Here's how the part is built. I have some questions about the finished solid (model axes, mm). A direction names the side the tool comes from. Round coordinates to 2 decimals unless told otherwise and drop trailing zeros. Write each loop counter-clockwise with the first axis right and the second up, starting at its lowest first coordinate (ties: lowest second). Pieces come first, ordered by that corner, then holes. Notation, with made-up numbers: (-15, 80) -> (10, 80) arc R20 ccw to (10, 107) -> close; hole circle Ø2 at (27.25, -31). An arc over 180 degrees is marked (long way). Answer as CSV lines item,"result".
from build123d import *

# Parameters (mm, degrees)
SKETCH1_W               = 1100
SKETCH1_H               = 670
BOSS_EXTRUDE1_DEPTH     = 15
SKETCH2_W               = 30
SKETCH2_H               = 30
BOSS_EXTRUDE2_DEPTH     = 725
MIRROR2_COPY_1_SKETCH_W = 30
MIRROR2_COPY_1_SKETCH_H = 30
MIRROR2_COPY_1_DEPTH    = 725
BOSS_EXTRUDE3_REACH     = 1112.808
SKETCH3_W               = 20
SKETCH3_H               = 40
BOSS_EXTRUDE4_REACH     = 1334.794
SKETCH4_W               = 20
SKETCH4_H               = 40


with BuildPart() as part:
    # Sketch1 → Boss-Extrude1 (new body)
    with BuildSketch(Plane(origin=(0, 0, 0), x_dir=(1, 0, 0), z_dir=(0, 1, 0))):
        Rectangle(SKETCH1_W, SKETCH1_H)
    extrude(amount=BOSS_EXTRUDE1_DEPTH)

    # Sketch2 → Boss-Extrude2 (add)
    with BuildSketch(Plane(origin=(0, 0, 0), x_dir=(1, 0, 0), z_dir=(0, 1, 0))):
        with Locations((-532, -317)):
            Rectangle(SKETCH2_W, SKETCH2_H)
    boss_extrude2 = extrude(amount=-BOSS_EXTRUDE2_DEPTH)

    # Mirror1: Boss-Extrude2 across plane
    add(boss_extrude2.mirror(Plane.XY))

    # Mirror2: Boss-Extrude2 across plane
    add(boss_extrude2.mirror(Plane(origin=(0, 0, 0), x_dir=(0, 0, 1), z_dir=(1, 0, 0))))

    # Mirror2 copy 1 sketch → Mirror2 copy 1 (add)
    with BuildSketch(Plane(origin=(0, 0, 0), x_dir=(-1, 0, 0), z_dir=(0, 1, 0))):
        with Locations((-532, -317)):
            Rectangle(MIRROR2_COPY_1_SKETCH_W, MIRROR2_COPY_1_SKETCH_H)
    extrude(amount=-MIRROR2_COPY_1_DEPTH)

    # Sketch3 → Boss-Extrude3 (add, up to next)
    with BuildSketch(Plane.XY.offset(-302), mode=Mode.PRIVATE) as boss_extrude3_sk1:
        with Locations((-527, -20)):
            Rectangle(SKETCH3_W, SKETCH3_H)
    boss_extrude3_tool1 = extrude(boss_extrude3_sk1.sketch, amount=BOSS_EXTRUDE3_REACH, mode=Mode.PRIVATE) - part.part
    boss_extrude3 = boss_extrude3_tool1.solids().sort_by_distance((-527, -20, -302))[0]
    add(boss_extrude3)

    # Mirror3: Boss-Extrude3 across plane
    add(boss_extrude3.mirror(Plane(origin=(0, 0, 0), x_dir=(0, 0, 1), z_dir=(1, 0, 0))))

    # Sketch4 → Boss-Extrude4 (add, up to next)
    with BuildSketch(Plane(origin=(-517, 0, 0), x_dir=(0, 0, -1), z_dir=(1, 0, 0)), mode=Mode.PRIVATE) as boss_extrude4_sk1:
        with Locations((-312, -20)):
            Rectangle(SKETCH4_W, SKETCH4_H)
    boss_extrude4_tool1 = extrude(boss_extrude4_sk1.sketch, amount=BOSS_EXTRUDE4_REACH, mode=Mode.PRIVATE) - part.part
    boss_extrude4 = boss_extrude4_tool1.solids().sort_by_distance((-517, -20, 312))[0]
    add(boss_extrude4)

    # Mirror4: Boss-Extrude4 across plane
    add(boss_extrude4.mirror(Plane.XY))


solid = part.part
Item 1: Suppose I cut it at B-B, the plane x = -186. List the corners of the cut face in (y, z) for me.
Results found:
outline,"(-40, -322) -> (0, -322) -> (0, -335) -> (15, -335) -> (15, 335) -> (0, 335) -> (0, 322) -> (-40, 322) -> (-40, 302) -> (0, 302) -> (0, -302) -> (-40, -302) -> close"
Item 2: If we mould it in two halves opening along X, with no side actions, what happens to faces 5 (the flat face through (-537, -20, -4)), 6 (the flat face through (-7, -20, -302)), 7 (the flat face through (532, -725, -317))? For each: pulls with the +X half, pulls with the -X half, needs draft (parallel to the pull), parting line crosses it, or undercut.
Results found:
face 5,"pulls with the -X half"
face 6,"undercut"
face 7,"needs draft"
Item 3: Suppose I cut it at A-A, the plane y = -139. List the corners of the cut face in (x, z) for me.
Results found:
outline,"(-547, -332) -> (-517, -332) -> (-517, -302) -> (-547, -302) -> close; (-547, 302) -> (-517, 302) -> (-517, 332) -> (-547, 332) -> close; (517, -332) -> (547, -332) -> (547, -302) -> (517, -302) -> close; (517, 302) -> (547, 302) -> (547, 332) -> (517, 332) -> close"
Item 4: Suppose I cut it at C-C, the plane z = 191.5. List the corners of the cut face in (x, y) for me.
Results found:
outline,"(-550, 0) -> (-537, 0) -> (-537, -40) -> (-517, -40) -> (-517, 0) -> (517, 0) -> (517, -40) -> (537, -40) -> (537, 0) -> (550, 0) -> (550, 15) -> (-550, 15) -> close"
Item 5: For faces 1 (the flat face through (-547, -357, 317)), 2 (the flat face through (532, -357, 332)), 3 (the flat face through (537, -20, -4)), 4 (the flat face through (-7, -20, 322)), which set-ups out of +Z, -Z, +X, -X, +Y, -Y let a thin tool reach every point of the face, with its end or its side?
Results found:
face 1,"+Z, -Z, -X, -Y"
face 2,"+Z, +X, -X, -Y"
face 3,"+X, -Y"
face 4,"+Z, -Y"
Item 6: Will these pins go through, and if not, where does the flat tip stop? pin 1 (12 mm diameter, centred on x = -233, y = -20.5, fed in from +Z); pin 2 (20 mm diameter, centred on y = -24.5, z = 72, fed in from -X); pin 3 (9 mm diameter, centred on x = -527, y = -516.5, fed in from -Z).
Results found:
pin 1,"stops at z = 322"
pin 2,"stops at x = -537"
pin 3,"stops at z = -332"
Item 7: I need wall thicknesses on L1, parallel to Z at x = 430.5, y = -19.5; L2, parallel to Y at x = 19, z = 98. Which ranges of each line are inside material? Lowest first, please.
Results found:
L1,"z = -322 to -302, 302 to 322"
L2,"y = 0 to 15"
